Verification items for the finished model (mm, model axes). Face numbers are marked on the shaded views. A direction names the side the tool comes from. Coordinates: 2 decimals unless noted, no trailing zeros. Write each loop counter-clockwise with the first axis right and the second up, starting at its lowest first coordinate (ties: lowest second). Pieces come first, ordered by that corner, then holes.
```python
from build123d import *

# Parameters (mm, degrees)
EXTRUDE_2_DEPTH     = 10
SKETCH_2_R          = 1.6
CUT_EXTRUDE_1_DEPTH = 10


with BuildPart() as part:
    # 草圖1 → 填料-伸長2 (new body)
    with BuildSketch(Plane.XY):
        with BuildLine():
            ThreePointArc((0, 55), (-2.5, 57.5), (-5, 55))
            Line((-5, 55), (-10, 27.5))
            Line((-10, 27.5), (-10, -5))
            Line((-10, -5), (-4.5, -13))
            ThreePointArc((-4.5, -13), (-3.667869554, -17.294945772), (-1.291902751, -20.968334127))
            Line((-1.291902751, -20.968334127), (-1.947985517, -23.157930655))
            Line((-1.947985517, -23.157930655), (-0.353660285, -24.365459974))
            Line((-0.353660285, -24.365459974), (1.576282518, -23.140674962))
            ThreePointArc((1.576282518, -23.140674962), (2.401767343, -23.540695254), (3.256508451, -23.873650308))
            Line((3.256508451, -23.873650308), (3.671596164, -26.12142248))
            Line((3.671596164, -26.12142248), (5.641228986, -26.468620617))
            Line((5.641228986, -26.468620617), (6.799870704, -24.498258488))
            ThreePointArc((6.799870704, -24.498258488), (7.716939899, -24.477630295), (8.629447558, -24.383975608))
            Line((8.629447558, -24.383975608), (10.024280034, -26.194837259))
            Line((10.024280034, -26.194837259), (11.935396246, -25.605231608))
            Line((11.935396246, -25.605231608), (12.067538645, -23.323277197))
            ThreePointArc((12.067538645, -23.323277197), (12.874201866, -22.886544009), (13.643490442, -22.386907624))
            Line((13.643490442, -22.386907624), (15.710846923, -23.362004916))
            Line((15.710846923, -23.362004916), (17.142510983, -21.965459886))
            Line((17.142510983, -21.965459886), (16.219048856, -19.874528216))
            ThreePointArc((16.219048856, -19.874528216), (16.737633381, -19.117883305), (17.194262154, -18.322313325))
            Line((17.194262154, -18.322313325), (19.478794182, -18.246874857))
            Line((19.478794182, -18.246874857), (20.115672942, -16.350988403))
            Line((20.115672942, -16.350988403), (18.340004717, -14.911620519))
            ThreePointArc((18.340004717, -14.911620519), (18.456288995, -14.001719757), (18.499682563, -13.085445547))
            Line((18.499682563, -13.085445547), (20.498207378, -11.976087123))
            Line((20.498207378, -11.976087123), (20.200024227, -9.998440337))
            Line((20.200024227, -9.998440337), (17.963252163, -9.527666203))
            ThreePointArc((17.963252163, -9.527666203), (17.651623839, -8.664921039), (17.272224493, -7.829757842))
            Line((17.272224493, -7.829757842), (18.544554248, -5.930822735))
            Line((18.544554248, -5.930822735), (17.376985928, -4.307004944))
            Line((17.376985928, -4.307004944), (15.171773349, -4.908515567))
            ThreePointArc((15.171773349, -4.908515567), (14.50087055, -4.28295113), (13.782243416, -3.712848971))
            Line((13.782243416, -3.712848971), (14.048139364, -1.442589758))
            Line((14.048139364, -1.442589758), (12.268350249, -0.530257194))
            Line((12.268350249, -0.530257194), (10.580409299, -2.07156602))
            ThreePointArc((10.580409299, -2.07156602), (8.812871925, -1.643790448), (7, -1.5))
            Line((7, -1.5), (0, 0))
            add(Edge.make_bspline(
                [(0, 55), (-10, 27.5), (0, 0)],
                knots=[0, 0, 0, 1, 1, 1], degree=2))
        make_face()
    extrude(amount=EXTRUDE_2_DEPTH)

    # 草圖2 → 除料-伸長1 (cut)
    with BuildSketch(Plane(origin=(0, 0, 0), x_dir=(-1, 0, 0), z_dir=(0, 0, -1))):
        with Locations((-7, -13)):
            Circle(SKETCH_2_R)
    extrude(amount=-CUT_EXTRUDE_1_DEPTH, mode=Mode.SUBTRACT)


solid = part.part
```
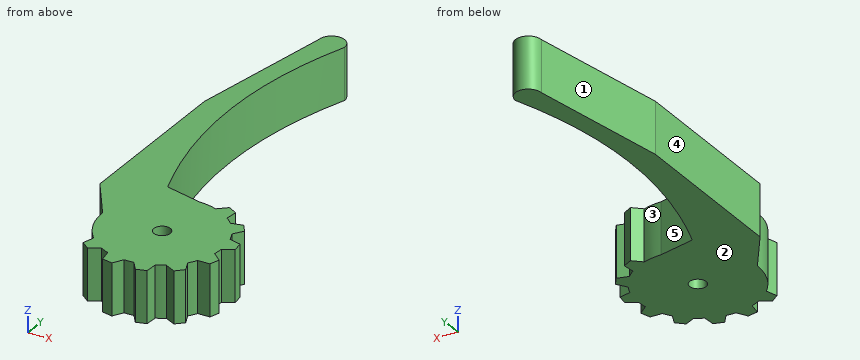
1. Draft check along X on the marked faces 1, 2 and 3. Enter one of: pulls with the +X half, pulls with the -X half, needs draft (parallel to the pull), parting line crosses it, or undercut.
2. Sectioned sample at A-A, the plane x = -7. Record the boundary of the cut face in (y, z), and give its area (3 significant figures).
3. Material ranges on L1, parallel to Y at x = 7, z = 5.75; L2, parallel to X at y = 23.5, z = 1.75; L3, parallel to Y at x = 18, z = 3.75, recorded low to high.
4. Tool access check on the marked faces 4 and 5. Record the directions out of +Z, -Z, +X, -X, +Y, -Y that give a thin tool (end or side, any length) a straight path to the whole face; none if there is none.
5. Gauge pin test, flat ends, axial feed: P1, Ø4, axis at x = 15.5, z = 7, coming from the -Y side; P2, Ø3, axis at y = 24, z = 1.5, coming from the +X side; P3, Ø1, axis at x = 12, z = 4, coming from the +Y side; P4, Ø2.5, axis at x = 7, y = -13, coming from the -Z side. Record the tip position at first contact, or that the pin passes through.
Outcome:
1. face 1: pulls with the -X half
1. face 2: needs draft
1. face 3: undercut
2. outline: (-9.36, 0) - (44, 0) - (44, 10) - (-9.36, 10) - close
2. area: 534 mm2
3. L1: y = -24.5 to -14.6, -11.4 to -1.5
3. L2: x = -10 to -4.89
3. L3: y = -18.3 to -9.54, -6.74 to -5.17
4. face 4: +Z, -Z, -X, +Y, -Y
4. face 5: +Z, -Z, +Y
5. P1: stops at y = -23.36
5. P2: stops at x = -4.83
5. P3: stops at y = -0.53
5. P4: passes through
